from build123d import *

# Parameters (mm, degrees)
F0_W      = 40
F0_H      = 10
F1_DEPTH  = 4
F2_R      = 1.25
F3_DEPTH  = 2.5
F4_DEPTH  = 0.7
F5_DEPTH  = 0.2
F6_DEPTH  = 0.5
F7_DEPTH  = 25
F9_DEPTH  = 0.5
F11_DEPTH = 0.5
F12_SIZE  = 0.2


with BuildPart() as f1:
    # F0 (on Top) → F1 (new body)
    with BuildSketch(Plane.XY):
        with Locations((0.5716348439, 33.2741251273)):
            Rectangle(F0_W, F0_H)
    extrude(amount=F1_DEPTH)

    # F2 (on face) → F3 (cut)
    with BuildSketch(Plane.XY.offset(4)):
        Polygon((-17.5513593567, 32.9373213533), (-15.2651689301, 30.6511309267), (-14.5890208517, 30.8323042582), (-14.6666665652, 31.1220820061), (-12.8959685214, 31.596539117), (-12.8183228079, 31.3067613691), (-12.1421747295, 31.4879347007), (-11.3053709554, 34.6109289013), (-13.591561382, 36.8971193279), (-16.7145555827, 36.0603155539), (-16.8957289142, 35.3841674755), (-16.6059511663, 35.3065217619), (-17.0804082772, 33.5358237181), (-17.3701860251, 33.6134694317), align=None)
        with Locations((-14.4283651561, 33.7741251273)):
            Circle(F2_R, mode=Mode.SUBTRACT)
        Polygon((-14.6666665652, 31.1220820061), (-14.5890208517, 30.8323042582), (-12.8183228079, 31.3067613691), (-12.8959685214, 31.596539117), align=None)
        Polygon((-16.8957289142, 35.3841674755), (-17.3701860251, 33.6134694317), (-17.0804082772, 33.5358237181), (-16.6059511663, 35.3065217619), align=None)
        Polygon((-7.6071271103, 32.9223784287), (-5.2801118546, 30.5953631731), (-4.6039637762, 30.7765365046), (-4.7074913943, 31.1629068352), (-2.8810255969, 31.6523068706), (-2.7774979788, 31.2659365401), (-2.1013499004, 31.4471098716), (-1.2496032019, 34.6258718258), (-3.5766184575, 36.9528870815), (-6.7553804117, 36.1011403829), (-6.9365537433, 35.4249923045), (-6.5501834128, 35.3214646865), (-7.0395834482, 33.4949988891), (-7.4259537787, 33.5985265071), align=None)
        with Locations((-4.4283651561, 33.7741251273)):
            Circle(F2_R, mode=Mode.SUBTRACT)
        Polygon((-4.7074913943, 31.1629068352), (-4.6039637762, 30.7765365046), (-2.7774979788, 31.2659365401), (-2.8810255969, 31.6523068706), align=None)
        Polygon((-6.9365537433, 35.4249923045), (-7.4259537787, 33.5985265071), (-7.0395834482, 33.4949988891), (-6.5501834128, 35.3214646865), align=None)
        Polygon((2.3928728897, 32.9223784287), (4.7198881454, 30.5953631731), (5.3960362238, 30.7765365046), (5.2925086057, 31.1629068352), (7.1189744031, 31.6523068706), (7.2225020212, 31.2659365401), (7.8986500996, 31.4471098716), (8.7503967981, 34.6258718258), (6.4233815425, 36.9528870815), (3.2446195883, 36.1011403829), (3.0634462567, 35.4249923045), (3.4498165872, 35.3214646865), (2.9604165518, 33.4949988891), (2.5740462213, 33.5985265071), align=None)
        with Locations((5.5716348439, 33.7741251273)):
            Circle(F2_R, mode=Mode.SUBTRACT)
        Polygon((3.0634462567, 35.4249923045), (2.5740462213, 33.5985265071), (2.9604165518, 33.4949988891), (3.4498165872, 35.3214646865), align=None)
        Polygon((5.2925086057, 31.1629068352), (5.3960362238, 30.7765365046), (7.2225020212, 31.2659365401), (7.1189744031, 31.6523068706), align=None)
        Polygon((12.3928728897, 32.9223784287), (14.7198881454, 30.5953631731), (15.3960362238, 30.7765365046), (15.2666267012, 31.2594994178), (17.0930924986, 31.7488994532), (17.2225020212, 31.2659365401), (17.8986500996, 31.4471098716), (18.7503967981, 34.6258718258), (16.4233815425, 36.9528870815), (13.2446195883, 36.1011403829), (13.0634462567, 35.4249923045), (13.5464091699, 35.295582782), (13.0570091345, 33.4691169846), (12.5740462213, 33.5985265071), align=None)
        with Locations((15.5716348439, 33.7741251273)):
            Circle(F2_R, mode=Mode.SUBTRACT)
        Polygon((15.2666267012, 31.2594994178), (15.3960362238, 30.7765365046), (17.2225020212, 31.2659365401), (17.0930924986, 31.7488994532), align=None)
        Polygon((13.0634462567, 35.4249923045), (12.5740462213, 33.5985265071), (13.0570091345, 33.4691169846), (13.5464091699, 35.295582782), align=None)
    extrude(amount=-F3_DEPTH, mode=Mode.SUBTRACT)

    # F2 (on face) → F4 (cut)
    with BuildSketch(Plane.XY.offset(4)):
        Polygon((-18.9036555135, 33.2996680164), (-17.5513593567, 32.9373213533), (-17.3701860251, 33.6134694317), (-18.0463341035, 33.7946427632), (-17.5718769926, 35.565340807), (-16.8957289142, 35.3841674755), (-16.7145555827, 36.0603155539), (-18.0668517395, 36.422662217), align=None)
        Polygon((-14.5890208517, 30.8323042582), (-15.2651689301, 30.6511309267), (-14.9028222669, 29.2988347699), (-11.7798280663, 30.1356385439), (-12.1421747295, 31.4879347007), (-12.8183228079, 31.3067613691), (-12.6371494763, 30.6306132907), (-14.4078475201, 30.1561561798), align=None)
        Polygon((-4.6039637762, 30.7765365046), (-5.2801118546, 30.5953631731), (-4.9177651915, 29.2430670163), (-1.7390032373, 30.0948137148), (-2.1013499004, 31.4471098716), (-2.7774979788, 31.2659365401), (-2.5963246472, 30.5897884617), (-4.4227904446, 30.1003884262), align=None)
        Polygon((-8.9594232671, 33.2847250919), (-7.6071271103, 32.9223784287), (-7.4259537787, 33.5985265071), (-8.1021018571, 33.7796998387), (-7.6127018217, 35.6061656361), (-6.9365537433, 35.4249923045), (-6.7553804117, 36.1011403829), (-8.1076765685, 36.4634870461), align=None)
        Polygon((1.0405767329, 33.2847250919), (2.3928728897, 32.9223784287), (2.5740462213, 33.5985265071), (1.8978981429, 33.7796998387), (2.3872981783, 35.6061656361), (3.0634462567, 35.4249923045), (3.2446195883, 36.1011403829), (1.8923234315, 36.4634870461), align=None)
        Polygon((5.3960362238, 30.7765365046), (4.7198881454, 30.5953631731), (5.0822348085, 29.2430670163), (8.2609967627, 30.0948137148), (7.8986500996, 31.4471098716), (7.2225020212, 31.2659365401), (7.4036753528, 30.5897884617), (5.5772095554, 30.1003884262), align=None)
        Polygon((15.3960362238, 30.7765365046), (14.7198881454, 30.5953631731), (15.0822348085, 29.2430670163), (18.2609967627, 30.0948137148), (17.8986500996, 31.4471098716), (17.2225020212, 31.2659365401), (17.4036753528, 30.5897884617), (15.5772095554, 30.1003884262), align=None)
        Polygon((11.0405767329, 33.2847250919), (12.3928728897, 32.9223784287), (12.5740462213, 33.5985265071), (11.8978981429, 33.7796998387), (12.3872981783, 35.6061656361), (13.0634462567, 35.4249923045), (13.2446195883, 36.1011403829), (11.8923234315, 36.4634870461), align=None)
    extrude(amount=-F4_DEPTH, mode=Mode.SUBTRACT)

    # F2 (on face) → F5 (join)
    with BuildSketch(Plane.XY.offset(4)):
        Polygon((-18.0463341035, 33.7946427632), (-17.3701860251, 33.6134694317), (-16.8957289142, 35.3841674755), (-17.5718769926, 35.565340807), align=None)
        Polygon((-12.8183228079, 31.3067613691), (-14.5890208517, 30.8323042582), (-14.4078475201, 30.1561561798), (-12.6371494763, 30.6306132907), align=None)
        Polygon((-2.7774979788, 31.2659365401), (-4.6039637762, 30.7765365046), (-4.4227904446, 30.1003884262), (-2.5963246472, 30.5897884617), align=None)
        Polygon((-8.1021018571, 33.7796998387), (-7.4259537787, 33.5985265071), (-6.9365537433, 35.4249923045), (-7.6127018217, 35.6061656361), align=None)
    extrude(amount=F5_DEPTH)

    # F2 (on face) → F6 (join)
    with BuildSketch(Plane.XY.offset(4)):
        Polygon((1.8978981429, 33.7796998387), (2.5740462213, 33.5985265071), (3.0634462567, 35.4249923045), (2.3872981783, 35.6061656361), align=None)
        Polygon((7.2225020212, 31.2659365401), (5.3960362238, 30.7765365046), (5.5772095554, 30.1003884262), (7.4036753528, 30.5897884617), align=None)
        Polygon((11.8978981429, 33.7796998387), (12.5740462213, 33.5985265071), (13.0634462567, 35.4249923045), (12.3872981783, 35.6061656361), align=None)
        Polygon((17.2225020212, 31.2659365401), (15.3960362238, 30.7765365046), (15.5772095554, 30.1003884262), (17.4036753528, 30.5897884617), align=None)
    extrude(amount=F6_DEPTH)

    # F7 (cut): faces of the model
    f7_faces = [f1.faces().sort_by_distance(p)[0] for p in [
        (-14.4283651561, 33.7741251273, 4),
        (-4.4283651561, 33.7741251273, 4),
        (5.5716348439, 33.7741251273, 4),
        (15.5716348439, 33.7741251273, 4),
    ]]
    extrude(f7_faces, amount=-F7_DEPTH, mode=Mode.SUBTRACT)

    # F8 (on face) → F9 (join)
    with BuildSketch(Plane.XY.offset(4.2)):
        Polygon((-17.5718769926, 35.565340807), (-18.0463341035, 33.7946427632), (-17.3701860251, 33.6134694317), (-16.8957289142, 35.3841674755), align=None)
        Polygon((-16.8957289142, 35.3841674755), (-17.3701860251, 33.6134694317), (-17.0804082772, 33.5358237181), (-16.6059511663, 35.3065217619), align=None)
        Polygon((-14.5890208517, 30.8323042582), (-14.4078475201, 30.1561561798), (-12.6371494763, 30.6306132907), (-12.8183228079, 31.3067613691), (-12.8959685214, 31.596539117), (-14.6666665652, 31.1220820061), align=None)
        Polygon((-7.6127018217, 35.6061656361), (-8.1021018571, 33.7796998387), (-7.4259537787, 33.5985265071), (-6.9365537433, 35.4249923045), align=None)
        Polygon((-6.9365537433, 35.4249923045), (-7.4259537787, 33.5985265071), (-6.9429908655, 33.4691169846), (-6.4535908301, 35.295582782), align=None)
        Polygon((-4.6039637762, 30.7765365046), (-4.4227904446, 30.1003884262), (-2.5963246472, 30.5897884617), (-2.7774979788, 31.2659365401), align=None)
        Polygon((-4.7333732988, 31.2594994178), (-4.6039637762, 30.7765365046), (-2.7774979788, 31.2659365401), (-2.9069075014, 31.7488994532), align=None)
    extrude(amount=F9_DEPTH)

    # F10 (on face) → F11 (join)
    with BuildSketch(Plane.XY.offset(4.5)):
        Polygon((2.3872981783, 35.6061656361), (1.8978981429, 33.7796998387), (2.5740462213, 33.5985265071), (3.0634462567, 35.4249923045), align=None)
        Polygon((3.0634462567, 35.4249923045), (2.5740462213, 33.5985265071), (2.8638239692, 33.5208807936), (3.3532240046, 35.347346591), align=None)
        Polygon((5.3960362238, 30.7765365046), (5.5772095554, 30.1003884262), (7.4036753528, 30.5897884617), (7.2225020212, 31.2659365401), align=None)
        Polygon((5.3183905103, 31.0663142525), (5.3960362238, 30.7765365046), (7.2225020212, 31.2659365401), (7.1448563077, 31.5557142879), align=None)
        Polygon((12.3872981783, 35.6061656361), (11.8978981429, 33.7796998387), (12.5740462213, 33.5985265071), (13.0634462567, 35.4249923045), align=None)
        Polygon((13.0634462567, 35.4249923045), (12.5740462213, 33.5985265071), (13.0570091345, 33.4691169846), (13.5464091699, 35.295582782), align=None)
        Polygon((15.3960362238, 30.7765365046), (15.5772095554, 30.1003884262), (17.4036753528, 30.5897884617), (17.2225020212, 31.2659365401), align=None)
        Polygon((15.2666267012, 31.2594994178), (15.3960362238, 30.7765365046), (17.2225020212, 31.2659365401), (17.0930924986, 31.7488994532), align=None)
    extrude(amount=F11_DEPTH)

    # F12
    f12_edges = [f1.edges().sort_by_distance(p)[0] for p in [
        (-16.84318, 34.421173, 4.7),
        (-13.781318, 31.359311, 4.7),
        (-6.698291, 34.38235, 4.7),
        (-3.82014, 31.504199, 4.7),
        (3.108524, 34.434114, 5),
        (6.231623, 31.311014, 5),
        (13.301709, 34.38235, 4.5),
        (16.17986, 31.504199, 5),
    ]]
    chamfer(f12_edges, length=F12_SIZE)


solid = f1.part
Geometry check sheet. Reference: the model listing, model coordinates, mm. A direction names the side the tool comes from. Round coordinates to 2 decimals unless told otherwise and drop trailing zeros. Write each loop counter-clockwise with the first axis right and the second up, starting at its lowest first coordinate (ties: lowest second). Pieces come first, ordered by that corner, then holes. Notation, with made-up numbers: (-9.5, -35.5) -> (-3.5, -35.5) arc R13 ccw to (-3.5, -21.5) -> close; hole circle Ø8 at (0, 1). An arc over 180 degrees is marked (long way). One line per item, written item: value. Start each with the question number.
(1) Go/stop test with flat-tipped pins: pin 1 Ø6 at (x, y) = (-6.5, 34) entering from +Z; pin 2 Ø1.9 at (x, y) = (-5, 32.5) entering from +Z; pin 3 Ø2 at (x, y) = (15.57, 33.77) entering from +Z. Record where each tip stops, or that it passes through.
(2) Cross-section at C-C, the plane z = 2.2. Record the cut outline in (x, y) (1 decimal), and give its area (3 significant figures).
(3) Scan lines: line 1 (X direction, y = 32.25, z = 3.2); line 2 (X direction, y = 33.25, z = 2.85); line 3 (Z direction, x = -3, y = 30.25). Record each from-to range of solid material in increasing order. Write a range as [from, to].
(4) Draft check along X on faces 6 (the flat face through (-13.6, 30.8, 4.7)), 7 (the flat face through (13.54, 31.775, 2.768)), 8 (the flat face through (20.572, 33, 2)). Enter one of: +X half, -X half, draft (parallel to the pull), parting line (faces both ways), or undercut.
(5) Cross-section at B-B, the plane y = 29.75. Record the cut outline in (x, z), and give its area (3 significant figures).
(6) Cross-section at A-A, the plane z = 0.7. Record the cut outline in (x, y).
(7) Access from +Z, -Z, +X, -X, +Y, -Y to the whole of each face (thin tool, end or side, straight path). Record for faces 1 (the flat face through (-8.528, 34.896, 3.655)), 2 (the flat face through (-4, 31, 4.7)), 3 (the flat face through (13, 35, 5)), 4 (the flat face through (-7, 34, 4.2)), 5 (the flat face through (0, 33, 0)).
Answer:
1. pin 1: z = 4.7
1. pin 2: z = 1.5
1. pin 3: through
2. outline: (-19.4, 28.3) -> (20.6, 28.3) -> (20.6, 38.3) -> (-19.4, 38.3) -> close; hole (-17.6, 32.9) -> (-15.3, 30.7) -> (-12.1, 31.5) -> (-11.3, 34.6) -> (-13.6, 36.9) -> (-16.7, 36.1) -> close; hole (-7.6, 32.9) -> (-5.3, 30.6) -> (-2.1, 31.4) -> (-1.2, 34.6) -> (-3.6, 37) -> (-6.8, 36.1) -> close; hole (2.4, 32.9) -> (4.7, 30.6) -> (7.9, 31.4) -> (8.8, 34.6) -> (6.4, 37) -> (3.2, 36.1) -> close; hole (12.4, 32.9) -> (14.7, 30.6) -> (17.9, 31.4) -> (18.8, 34.6) -> (16.4, 37) -> (13.2, 36.1) -> close
2. area: 288 mm²
3. line 1: [-19.43, -16.86], [-11.94, -6.93], [-1.89, 3.07], [8.11, 13.07], [18.11, 20.57]
3. line 2: [-19.43, -17.47], [-11.67, -7.52], [-1.62, 2.48], [8.38, 12.48], [18.38, 20.57]
3. line 3: [0, 3.3]
4. face 6: draft
4. face 7: undercut
4. face 8: +X half
5. outline: (-19.43, 0) -> (20.57, 0) -> (20.57, 4) -> (16.97, 4) -> (16.97, 3.3) -> (14.95, 3.3) -> (14.95, 4) -> (6.97, 4) -> (6.97, 3.3) -> (4.95, 3.3) -> (4.95, 4) -> (-3.03, 4) -> (-3.03, 3.3) -> (-5.05, 3.3) -> (-5.05, 4) -> (-13.22, 4) -> (-13.22, 3.3) -> (-15.02, 3.3) -> (-15.02, 4) -> (-19.43, 4) -> close
5. area: 154 mm²
6. outline: (-19.43, 28.27) -> (20.57, 28.27) -> (20.57, 38.27) -> (-19.43, 38.27) -> close; hole circle Ø2.5 at (-14.43, 33.77); hole circle Ø2.5 at (-4.43, 33.77); hole circle Ø2.5 at (5.57, 33.77); hole circle Ø2.5 at (15.57, 33.77)
7. face 1: +Z
7. face 2: +Z, -X, +Y, -Y
7. face 3: +Z, +X, -X, +Y, -Y
7. face 4: -Y
7. face 5: -Z, +X, -X, +Y, -Y
